For this review, take the finished solid that the model builds, in its own axes (mm). A direction names the side the tool comes from. Give positions to 0.01 mm unless a question says otherwise; leave off trailing zeros. Order: outer loops, then holes, each group sorted by start corner. A loop starts at its lowest first (then second) coordinate and runs counter-clockwise, first axis right, second up. Notation, with made-up numbers: (63.5, -16.75) - (92.5, -16.75) arc R9 cw to (92.5, -8.75) - close; hole circle Ø10 at (40, -20.5). An arc over 180 degrees is marked (long way). One line per item, written item: value.
```python
from build123d import *

# Parameters (mm, degrees)
SKETCH_1_R          = 12
EXTRUDE_1_DEPTH     = 18.4
SKETCH_2_R          = 9.9
EXTRUDE_2_DEPTH     = 4
EXTRUDE_START       = 4
SKETCH_3_R          = 9.9
EXTRUDE_3_DEPTH     = 4
EXTRUDE_4_DEPTH     = 15
SKETCH_4_R          = 2.1
CUT_EXTRUDE_1_DEPTH = 33.649042948


with BuildPart() as part:
    # 草图1 → 凸台-拉伸1 (new body)
    with BuildSketch(Plane.XY):
        Circle(SKETCH_1_R)
    extrude(amount=EXTRUDE_1_DEPTH)

    # 草图2 → 凸台-拉伸2 (add)
    with BuildSketch(Plane.XY.offset(18.4)):
        Circle(SKETCH_2_R)
    extrude(amount=EXTRUDE_2_DEPTH)

    # 草图3 → 凸台-拉伸3 (add)
    with BuildSketch(Plane(origin=(0, 0, 0), x_dir=(-1, 0, 0), z_dir=(0, 0, -1)).offset(EXTRUDE_START)):
        with Locations(Location((0, 0, 0), (0, 0, 180))):
            Circle(SKETCH_3_R)
    extrude(amount=-EXTRUDE_3_DEPTH)

    # 草图7 → 凸台-拉伸4 (add)
    with BuildSketch(Plane(origin=(0, 0, 0), x_dir=(0, 0, -1), z_dir=(1, 0, 0))):
        with BuildLine():
            Line((-12.154769624, 4.033526555), (-12.60491347, 1.574386356))
            add(Edge.make_bspline(
                [(-12.60491347, 1.574386356), (-16.365153372, -3), (-9.2, -3), (-2.034846628, -3), (-5.79508653, 1.574386356)],
                knots=[2.589117856, 2.589117856, 2.589117856, 4.71238898, 4.71238898, 6.835660105, 6.835660105, 6.835660105], degree=2, weights=[1, 0.487444637, 1, 0.487444637, 1]))
            Line((-5.79508653, 1.574386356), (-6.245230376, 4.033526555))
            Line((-6.245230376, 4.033526555), (-8.5, 2.9537053))
            add(Edge.make_bspline(
                [(-8.5, 2.9537053), (-9.2, 3.047020297), (-9.9, 2.9537053)],
                knots=[1.394890559, 1.394890559, 1.394890559, 1.746702095, 1.746702095, 1.746702095], degree=2, weights=[1, 0.984568433, 1]))
            Line((-9.9, 2.9537053), (-12.154769624, 4.033526555))
        make_face()
    extrude(amount=EXTRUDE_4_DEPTH)

    # 草图4 → 切除-拉伸1 (cut, through all)
    with BuildSketch(Plane.XY.offset(22.4)):
        with Locations((0, 6)):
            Circle(SKETCH_4_R)
        with Locations((6, 0)):
            Circle(SKETCH_4_R)
        with Locations((0, -6)):
            Circle(SKETCH_4_R)
        with Locations((-6, 0)):
            Circle(SKETCH_4_R)
    extrude(amount=-CUT_EXTRUDE_1_DEPTH, mode=Mode.SUBTRACT)


solid = part.part
```
(1) For P1, Ø6.5, axis at x = 0, y = -6, coming from the -Z side; P2, Ø3.5, axis at x = 6, y = 0, coming from the -Z side; P3, Ø4, axis at y = 5, z = 8.5, coming from the -X side; P4, Ø4, axis at y = -5.5, z = 12.5, coming from the -X side, all flat-tipped, find the tip position at first contact; note any pin that passes through.
Answers below:
P1: stops at z = -4
P2: passes through
P3: stops at x = -11.62
P4: stops at x = -11.48
(2) Take a section at A-A (x = 0). Write out the cut boundary in (y, z).
Answers below:
outline: (-12, 0) - (-9.9, 0) - (-9.9, -4) - (-8.1, -4) - (-8.1, 22.4) - (-9.9, 22.4) - (-9.9, 18.4) - (-12, 18.4) - close; (-3.9, -4) - (3.9, -4) - (3.9, 22.4) - (-3.9, 22.4) - close; (8.1, -4) - (9.9, -4) - (9.9, 0) - (12, 0) - (12, 18.4) - (9.9, 18.4) - (9.9, 22.4) - (8.1, 22.4) - close
(3) Draft analysis for pull direction X (two halves, no side actions). For faces 4 (the face through (-0.46, -8.05, 9.38)), 5 (the face through (9.443, 2.974, 20.372)), 6 (the face through (0, 0, -4)), state which applies: pulls with the +X half, pulls with the -X half, needs draft (parallel to the pull), parting line crosses it, or undercut.
Answers below:
face 4: undercut
face 5: parting line crosses it
face 6: needs draft
(4) Machinability: for faces 1 (the face through (13.125, 2.821, 12.377)), 2 (the face through (13.13, 3.5, 7.36)), 3 (the face through (13.125, 2.787, 6.017)), which of the approach directions +Z, -Z, +X, -X, +Y, -Y give a long, thin tool a straight path to every point of the face, cutting with its end or side? Answer none if there is none.
Answers below:
face 1: +Z, +X, +Y
face 2: +X, +Y
face 3: -Z, +X, +Y
(5) Wall thickness on line 1 (Y direction, x = -1.25, z = 10.5); line 2 (X direction, y = -1.75, z = 19); line 3 (X direction, y = 1.75, z = 16.75): over which ranges is each line inside the solid? List them lowest first. Write a range as from..to.
Answers below:
line 1: y = -11.93..-7.69, -4.31..4.31, 7.69..11.93
line 2: x = -9.74..-7.16, -4.84..4.84, 7.16..9.74
line 3: x = -11.87..-7.16, -4.84..4.84, 7.16..11.87
(6) Take a section at B-B (z = 2.5). Write out the cut boundary in (x, y).
Answers below:
outline: circle Ø24 at (0, 0); hole circle Ø4.2 at (-6, 0); hole circle Ø4.2 at (0, -6); hole circle Ø4.2 at (0, 6); hole circle Ø4.2 at (6, 0)
(7) Take a section at C-C (y = 6). Write out the cut boundary in (x, z), then the cut area to 3 significant figures.
Answers below:
outline: (-10.39, 0) - (-7.87, 0) - (-7.87, -4) - (-2.1, -4) - (-2.1, 22.4) - (-7.87, 22.4) - (-7.87, 18.4) - (-10.39, 18.4) - close; (2.1, -4) - (7.87, -4) - (7.87, 0) - (10.39, 0) - (10.39, 18.4) - (7.87, 18.4) - (7.87, 22.4) - (2.1, 22.4) - close
area: 398 mm^2
